from build123d import *

# Parameters (mm, degrees)
SKETCH1_W           = 42
SKETCH1_H           = 16
BOSS_EXTRUDE1_DEPTH = 7
SKETCH2_R           = 1.6
BOSS_EXTRUDE2_DEPTH = 1.6
CUT_EXTRUDE1_REACH  = 26.062
SKETCH3_R           = 1.45
SKETCH4_R           = 2.75
BOSS_EXTRUDE3_DEPTH = 3
BOSS_EXTRUDE4_DEPTH = 8
BOSS_EXTRUDE5_DEPTH = 3


with BuildPart() as part:
    # Sketch1 → Boss-Extrude1 (new body)
    with BuildSketch(Plane(origin=(0, 0, 0), x_dir=(1, 0, 0), z_dir=(0, 1, 0))):
        Rectangle(SKETCH1_W, SKETCH1_H)
    extrude(amount=BOSS_EXTRUDE1_DEPTH)

    # Sketch2 → Boss-Extrude2 (add)
    with BuildSketch(Plane(origin=(0, 7, 0), x_dir=(1, 0, 0), z_dir=(0, 1, 0))):
        with Locations(Location((-17, 5, 0), (0, 0, 270))):
            Circle(SKETCH2_R)
        with Locations(Location((-17, -5, 0), (0, 0, 270))):
            Circle(SKETCH2_R)
    extrude(amount=BOSS_EXTRUDE2_DEPTH)

    # Sketch3 → Cut-Extrude1 (cut, up to next)
    with BuildSketch(Plane(origin=(0, 0, 0), x_dir=(1, 0, 0), z_dir=(0, 1, 0)), mode=Mode.PRIVATE) as cut_extrude1_sk1:
        with Locations(Location((-2.5, 5, 0), (0, 0, 270))):
            Circle(SKETCH3_R)
    cut_extrude1_tool1 = extrude(cut_extrude1_sk1.sketch, amount=CUT_EXTRUDE1_REACH, mode=Mode.PRIVATE) & part.part
    # Sketch3 → Cut-Extrude1 (cut, up to next)
    with BuildSketch(Plane(origin=(0, 0, 0), x_dir=(1, 0, 0), z_dir=(0, 1, 0)), mode=Mode.PRIVATE) as cut_extrude1_sk2:
        with Locations(Location((17, 5, 0), (0, 0, 270))):
            Circle(SKETCH3_R)
    cut_extrude1_tool2 = extrude(cut_extrude1_sk2.sketch, amount=CUT_EXTRUDE1_REACH, mode=Mode.PRIVATE) & part.part
    add(cut_extrude1_tool1.solids().sort_by_distance((-2.5, 0, -5))[0], mode=Mode.SUBTRACT)
    add(cut_extrude1_tool2.solids().sort_by_distance((17, 0, -5))[0], mode=Mode.SUBTRACT)

    # Sketch4 → Boss-Extrude3 (add)
    # profile 1 of 2: a face of its own
    with BuildSketch(Plane(origin=(0, 0, 0), x_dir=(1, 0, 0), z_dir=(0, 1, 0))):
        with BuildLine():
            Line((12.854829477, 23.59812982), (5, 8))
            Line((5, 8), (35, 8))
            Line((35, 8), (27.145170523, 23.59812982))
            ThreePointArc((27.145170523, 23.59812982), (20, 28), (12.854829477, 23.59812982))
        make_face()
        with Locations(Location((20, 20, 0), (0, 0, 270))):
            Circle(SKETCH4_R, mode=Mode.SUBTRACT)
    # profile 2 of 2: a face of its own
    with BuildSketch(Plane(origin=(0, 0, 0), x_dir=(1, 0, 0), z_dir=(0, 1, 0))):
        with BuildLine():
            Line((35, -8), (27.145170523, -23.59812982))
            ThreePointArc((27.145170523, -23.59812982), (20, -28), (12.854829477, -23.59812982))
            Line((12.854829477, -23.59812982), (5, -8))
            Line((5, -8), (35, -8))
        make_face()
        with Locations(Location((20, -20, 0), (0, 0, 90))):
            Circle(SKETCH4_R, mode=Mode.SUBTRACT)
    extrude(amount=BOSS_EXTRUDE3_DEPTH)

    # Sketch5 → Boss-Extrude4 (add, symmetric)
    with BuildSketch(Plane.XY):
        Polygon((21, 7), (35, 3), (35, 0), (21, 0), align=None)
    extrude(amount=BOSS_EXTRUDE4_DEPTH, both=True)

    # Sketch6 → Boss-Extrude5 (add)
    with BuildSketch(Plane(origin=(0, 0, 0), x_dir=(1, 0, 0), z_dir=(0, 1, 0))):
        Polygon((35, -8), (44, -8), (44, 8), (39, 8), (39, 5), (41, 5), (41, -4), (35, -4), align=None)
    extrude(amount=BOSS_EXTRUDE5_DEPTH)


solid = part.part
Build history of the part. All positions in model axes, mm. A direction names the side the tool comes from. Give positions to 0.01 mm unless a question says otherwise; leave off trailing zeros. Loops run counter-clockwise (first coordinate to the right, second up) from the corner with the lowest first, then second, coordinate; pieces in that order, holes last. Notation, with made-up numbers: (36, -38) - (44, -38) arc R8 cw to (44, -31) - close; hole circle Ø6 at (32.5, -1.5). An arc over 180 degrees is marked (long way). Write item = value, one per line. Start each with the question number.
1) Drop flat-ended pins along their axis: pin 1 Ø1.5 at (x, z) = (-6.5, 1.5) entering from -Y; pin 2 Ø5 at (x, y) = (29, 3.5) entering from -Z; pin 3 Ø2.5 at (x, z) = (-2.5, -5) entering from +Y; pin 4 Ø1.5 at (x, y) = (40, 1) entering from +Z. Give the stop position or say it passes through.
2) Band-saw the part on A-A on x = -2.5. Give the cut face in (y, z), plus the area to 3 significant figures.
3) Band-saw the part on D-D on x = -17. Give the cut face in (y, z), plus the area to 3 significant figures.
4) Tool access for faces 1 (the flat face through (1, 4, 8)), 2 (the flat face through (35, 2, -2)), 3 (the flat face through (20, 3, -16)): list every direction of +Z, -Z, +X, -X, +Y, -Y with a clear straight run to the whole face (end or side of a thin tool).
5) Pull direction X, two halves, no side cores. Call faces 4 (the flat face through (44, 1, 0)), 5 (the cylindrical face through (16.12, 3.45, -6.15)), 6 (the flat face through (20, 3, 16)): +X half, -X half, draft (parallel to the pull), parting line (faces both ways), or undercut.
6) Band-saw the part on C-C on z = -1.5. Give the cut face in (x, y).
7) Probe probe 1 along X at (y, z) = (2, -6); probe 2 along Z at (x, y) = (17, 3.25); probe 3 along Z at (x, y) = (-15.5, 1.5). List the from-to ranges inside material, lowest first. Write a range as from..to.
8) Band-saw the part on B-B on y = 2. Give the cut face in (x, z), plus the area to 3 significant figures.
Final values:
q1.pin_1 = 0
q1.pin_2 = -24.59
q1.pin_3 = through
q1.pin_4 = 8
q2.outline = (0, -8) - (7, -8) - (7, -6.45) - (0, -6.45) - close; (0, -3.55) - (7, -3.55) - (7, 8) - (0, 8) - close
q2.area = 91.7 mm²
q3.outline = (0, -8) - (7, -8) - (7, -6.6) - (8.6, -6.6) - (8.6, -3.4) - (7, -3.4) - (7, 3.4) - (8.6, 3.4) - (8.6, 6.6) - (7, 6.6) - (7, 8) - (0, 8) - close
q3.area = 122 mm²
q4.face_1 = +Z, -X, +Y
q4.face_2 = -Z, +Y, -Y
q4.face_3 = -Z, +X, -X, +Y
q5.face_4 = +X half
q5.face_5 = undercut
q5.face_6 = draft
q6.outline = (-21, 0) - (35, 0) - (35, 3) - (21, 7) - (-21, 7) - close; (41, 0) - (44, 0) - (44, 3) - (41, 3) - close
q7.probe_1 = -21..-3.55, -1.45..15.95, 18.05..35, 39..44
q7.probe_2 = -8..-6.45, -3.55..8
q7.probe_3 = -8..8
q8.outline = (-21, -8) - (5, -8) - (12.85, -23.6) arc R8 ccw to (27.15, -23.6) - (35, -8) - (35, 4) - (41, 4) - (41, -5) - (39, -5) - (39, -8) - (44, -8) - (44, 8) - (35, 8) - (27.15, 23.6) arc R8 ccw to (12.85, 23.6) - (5, 8) - (-21, 8) - close; hole circle Ø2.9 at (-2.5, -5); hole circle Ø2.9 at (17, -5); hole circle Ø5.5 at (20, -20); hole circle Ø5.5 at (20, 20)
q8.area = 1,690 mm²
